```python
from build123d import *

# Parameters (mm, degrees)
SKETCH1_R           = 6.4
BOSS_EXTRUDE1_DEPTH = 7.45
SKETCH2_R           = 3.775
BOSS_EXTRUDE2_DEPTH = 100
CUT_EXTRUDE1_DEPTH  = 5
FILLET2_R           = 0.5
FILLET3_R           = 0.5


with BuildPart() as part:
    # Sketch1 → Boss-Extrude1 (new body)
    with BuildSketch(Plane(origin=(0, 0, 0), x_dir=(1, 0, 0), z_dir=(0, 1, 0))):
        Circle(SKETCH1_R)
    extrude(amount=BOSS_EXTRUDE1_DEPTH)

    # Sketch2 → Boss-Extrude2 (add)
    with BuildSketch(Plane(origin=(0, 7.45, 0), x_dir=(1, 0, 0), z_dir=(0, 1, 0))):
        Circle(SKETCH2_R)
    extrude(amount=BOSS_EXTRUDE2_DEPTH)

    # Sketch3 → Cut-Extrude1 (cut)
    with BuildSketch(Plane.XZ):
        Polygon((-3.608439182, 0), (-1.804219591, -3.125), (1.804219591, -3.125), (3.608439182, 0), (1.804219591, 3.125), (-1.804219591, 3.125), align=None)
    extrude(amount=-CUT_EXTRUDE1_DEPTH, mode=Mode.SUBTRACT)

    # Fillet2
    fillet2_edges = [part.edges().sort_by_distance(p)[0] for p in [
        (-2.706329387, 0, 1.5625),
        (-2.706329387, 0, -1.5625),
        (0, 0, -3.125),
        (2.706329387, 0, -1.5625),
        (2.706329387, 0, 1.5625),
        (0, 0, 3.125),
    ]]
    fillet(fillet2_edges, radius=FILLET2_R)

    # Fillet3
    fillet3_edges = [part.edges().sort_by_distance(p)[0] for p in [
        (-2.706329387, 5, 1.5625),
        (0, 5, 3.125),
        (2.706329387, 5, 1.5625),
        (2.706329387, 5, -1.5625),
        (0, 5, -3.125),
        (-2.706329387, 5, -1.5625),
    ]]
    fillet(fillet3_edges, radius=FILLET3_R)


solid = part.part
```
CAD build for the part. Positions are in the model's coordinates, mm. A direction names the side the tool comes from. Round coordinates to 2 decimals unless told otherwise and drop trailing zeros. Order: outer loops, then holes, each group sorted by start corner. A loop starts at its lowest first (then second) coordinate and runs counter-clockwise, first axis right, second up. Notation, with made-up numbers: (26, -27.75) - (45, -27.75) arc R28 ccw to (45, -0.75) - close; hole circle Ø10 at (-16, -14). An arc over 180 degrees is marked (long way). Answer in a Markdown table with one row per item. Add a question column.
(1) Band-saw the part on B-B on y = 11. List the corners of the cut face in (x, z) (3 decimals).
(2) Drop flat-ended pins along their axis: pin 1 Ø4 at (x, z) = (-1, 0) entering from -Y; pin 2 Ø4 at (x, y) = (0.5, 2) entering from +Z; pin 3 Ø1 at (x, y) = (-0.5, 41.5) entering from +Z (3 decimals); pin 4 Ø4 at (x, y) = (4, 20) entering from +Z. Give the stop position or say it passes through.
(3) Band-saw the part on A-A on x = 0. List the corners of the cut face in (y, z) (3 decimals), and give its area (3 significant figures).
(4) Probe L1, parallel to Y at x = -0.25, z = 1.5; L2, parallel to Y at x = -4.75, z = 0.5; L3, parallel to Z at x = -1, y = 14.5. List the from-to ranges inside material, lowest first. Write a range as [from, to].
(5) Mould opens along Z. For faces 4 (the face through (-5.08, 3.67, 3.89)), 5 (the face through (3, 7.45, 3)), 6 (the face through (2.595, 4.85, -1.469)) say: +Z half, -Z half, draft (parallel to the pull), parting line (faces both ways), or undercut.
(6) 3-axis set-ups, long thin cutter, end or side, ignore diameter. For faces 1 (the face through (0, 2, 3.125)), 2 (the face through (0, 107.45, 0)), 3 (the face through (-0.818, 56.75, 3.685)): which of +Z, -Z, +X, -X, +Y, -Y reach the whole face in a straight line?
(7) Band-saw the part on C-C on z = 5. List the corners of the cut face in (x, y) (3 decimals), and give its area (3 significant figures).
Data:
| question | item | result |
|---|---|---|
| 1 | outline | circle Ø7.55 at (0, 0) |
| 2 | pin 1 | stops at y = 4.94 |
| 2 | pin 2 | stops at z = 6.4 |
| 2 | pin 3 | stops at z = 3.775 |
| 2 | pin 4 | stops at z = 3.2 |
| 3 | outline | (0, -6.4) - (7.45, -6.4) - (7.45, -3.775) - (107.45, -3.775) - (107.45, 3.775) - (7.45, 3.775) - (7.45, 6.4) - (0, 6.4) - (0, 3.625) arc R0.5 ccw to (0.5, 3.125) - (4.5, 3.125) arc R0.5 cw to (5, 2.625) - (5, -2.625) arc R0.5 cw to (4.5, -3.125) - (0.5, -3.125) arc R0.5 ccw to (0, -3.625) - close |
| 3 | area | 819 mm^2 |
| 4 | L1 | y = [5, 107.45] |
| 4 | L2 | y = [0, 7.45] |
| 4 | L3 | z = [-3.64, 3.64] |
| 5 | face 4 | parting line |
| 5 | face 5 | draft |
| 5 | face 6 | undercut |
| 6 | face 1 | -Y |
| 6 | face 2 | +Z, -Z, +X, -X, +Y |
| 6 | face 3 | +Y |
| 7 | outline | (-3.995, 0) - (3.995, 0) - (3.995, 7.45) - (-3.995, 7.45) - close |
| 7 | area | 59.5 mm^2 |
